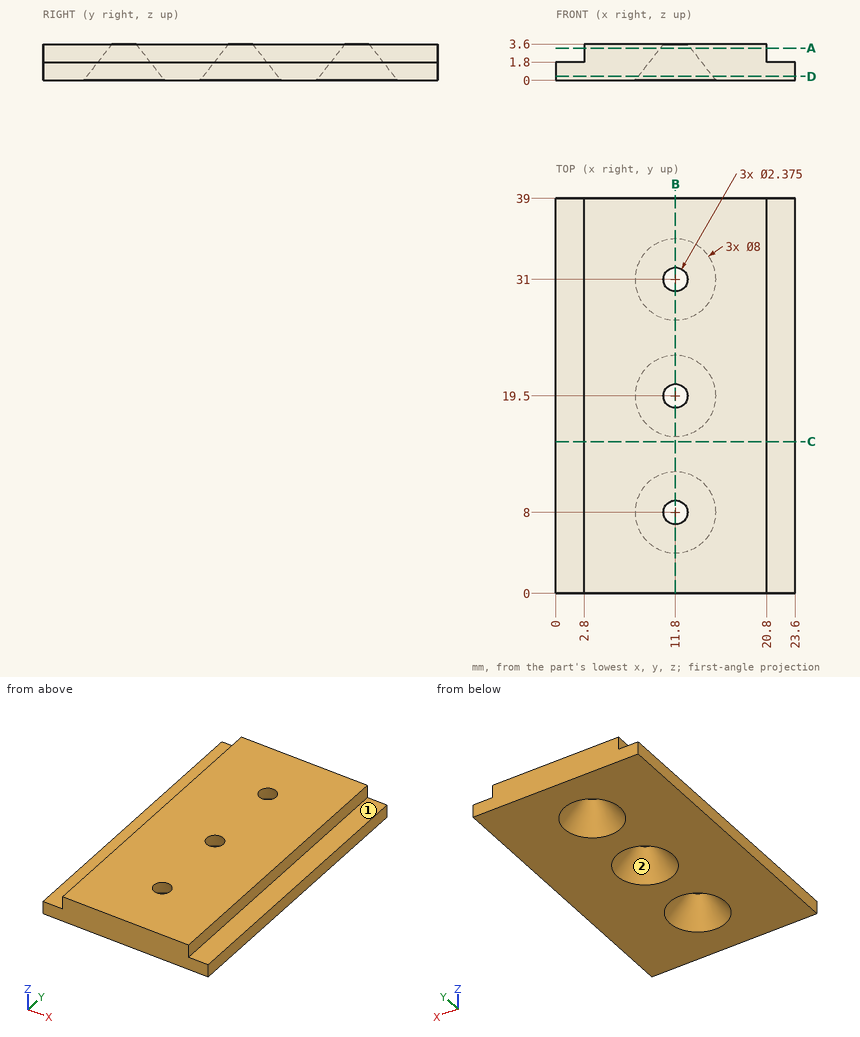
Job drawing, mm, ordinate dimensions from the low corner. One solid piece. Coordinates: 2 decimals unless noted, no trailing zeros. Order: outer loops, then holes, each group sorted by start corner. A loop starts at its lowest first (then second) coordinate and runs counter-clockwise, first axis right, second up. Notation, with made-up numbers: M 73,28.25 L 126,28.25 A8 cw 126,34.25 Z; hole C -17,85.5 d7. An arc over 180 degrees is marked long. Answer as CSV lines item,"result".
(1) Flat gauge pins, fed straight in: pin 1 (1 mm diameter, centred on y = 6, z = 2.5, fed in from +X); pin 2 (1.4 mm diameter, centred on x = 1, y = 16.5, fed in from +Z); pin 3 (1.5 mm diameter, centred on y = 31.5, z = 2.5, fed in from +X); pin 4 (2 mm diameter, centred on y = 26, z = 3, fed in from -X). Where does each tip first touch, or does it go through?
Geometry says:
pin 1,"stops at x = 20.8"
pin 2,"stops at z = 1.8"
pin 3,"stops at x = 23.6"
pin 4,"stops at x = 2.8"
(2) Band-saw the part on C-C, the plane y = 15. List the corners of the cut face in (x, z), then the cut area to 3 significant figures.
Geometry says:
outline,"M 0,0 L 23.6,0 L 23.6,1.8 L 20.8,1.8 L 20.8,3.6 L 2.8,3.6 L 2.8,1.8 L 0,1.8 Z"
area,"74.9 mm2"
(3) Wall check: line 1 along Y through (x, z) = (12.75, 0.95) (1 decimal); line 2 along X through (y, z) = (5.5, 3); line 3 along X through (y, z) = (29, 0.4). Give the ranges that are in metal, low to high.
Geometry says:
line 1,"y = 0 to 4.9, 11.1 to 16.4, 22.6 to 27.9, 34.1 to 39"
line 2,"x = 2.8 to 20.8"
line 3,"x = 0 to 8.7, 14.9 to 23.6"
(4) Band-saw the part on D-D, the plane z = 0.4. List the corners of the cut face in (x, y) (1 decimal).
Geometry says:
outline,"M 0,0 L 23.6,0 L 23.6,39 L 0,39 Z; hole C 11.8,8 d7.4; hole C 11.8,19.5 d7.4; hole C 11.8,31 d7.4"
(5) Pull direction X, two halves, no side cores. Call the marked faces 1 and 2: +X half, -X half, draft (parallel to the pull), parting line (faces both ways), or undercut.
Geometry says:
face 1,"draft"
face 2,"undercut"
(6) Band-saw the part on B-B, the plane x = 11.8. List the corners of the cut face in (y, z).
Geometry says:
outline,"M 0,0 L 4,0 L 6.81,3.6 L 0,3.6 Z; M 9.19,3.6 L 12,0 L 15.5,0 L 18.31,3.6 Z; M 20.69,3.6 L 23.5,0 L 27,0 L 29.81,3.6 Z; M 32.19,3.6 L 35,0 L 39,0 L 39,3.6 Z"
(7) Band-saw the part on A-A, the plane z = 3.2. List the corners of the cut face in (x, y).
Geometry says:
outline,"M 2.8,0 L 20.8,0 L 20.8,39 L 2.8,39 Z; hole C 11.8,8 d3; hole C 11.8,19.5 d3; hole C 11.8,31 d3"
